Part model, mm, in its own coordinate system. Face numbers are marked on the shaded views. A direction names the side the tool comes from. Give positions to 0.01 mm unless a question says otherwise; leave off trailing zeros. Write each loop counter-clockwise with the first axis right and the second up, starting at its lowest first coordinate (ties: lowest second). Pieces come first, ordered by that corner, then holes. Notation, with made-up numbers: (8.5, 56.25) - (22.5, 56.25) arc R16 ccw to (22.5, 69.25) - close; hole circle Ø10 at (-18, 9.5). An arc over 180 degrees is marked (long way). Answer in a Markdown table with one row per item. Add a question column.
1. Band-saw the part on B-B on x = -50.5. Write the cut outline in (y, z).
2. Band-saw the part on A-A on z = 4.2. State how many separate pieces and enclosed holes the cut face has, plus the area to 3 significant figures.
3. Probe line 1 along X through (y, z) = (45.5, 4.55); line 2 along Y through (x, z) = (-48.5, 2.4); line 3 along X through (y, z) = (34.25, 3.75). List the from-to ranges inside material, lowest first.
4. Drop flat-ended pins along their axis: pin 1 Ø2 at (y, z) = (30, 3) entering from -X; pin 2 Ø1.7 at (y, z) = (36, 2.5) entering from -X; pin 3 Ø1.8 at (x, z) = (-39, 2.5) entering from -Y. Give the stop position or say it passes through.
5. Pull direction Y, two halves, no side cores. Call the marked faces 5, 6 and 7: released by +Y, released by -Y, zero draft, split by the parting line, or undercut.
6. Band-saw the part on C-C on y = 44.5. Write the cut outline in (x, z).
7. Which spindle directions (+Z, -Z, +X, -X, +Y, -Y) get a long thin tool onto all of the face, cutting with end or side? Do the marked faces 1, 2, 3 and 4. Say none if no direction does.
8. Band-saw the part on D-D on x = -62. Write the cut outline in (y, z).
```python
from build123d import *

# Parameters (mm, degrees)
SKETCH2_W           = 40
SKETCH2_H           = 5
SKETCH2_R           = 10
BOSS_EXTRUDE2_DEPTH = 6
FILLET1_R           = 1
FILLET2_R           = 1
FILLET3_R           = 1


with BuildPart() as part:
    # Sketch2 → Boss-Extrude2 (new body)
    # profile 1 of 3: a face of its own
    with BuildSketch(Plane.XY):
        with BuildLine():
            ThreePointArc((-64.563103681, 49.969328221), (-53.382763794, 24.969328221), (-42.202423906, 49.969328221))
            Line((-42.202423906, 49.969328221), (-53.382763794, 49.969328221))
            Line((-53.382763794, 49.969328221), (-64.563103681, 49.969328221))
        make_face()
        with BuildLine():
            ThreePointArc((-43.382763794, 39.969328221), (-60.453831606, 32.89826041), (-53.382763794, 49.969328221))
            ThreePointArc((-53.382763794, 49.969328221), (-46.311695982, 47.040396033), (-43.382763794, 39.969328221))
        make_face(mode=Mode.SUBTRACT)
    # profile 2 of 3: a face of its own
    with BuildSketch(Plane.XY):
        with Locations((-53.382763794, 52.469328221)):
            Rectangle(SKETCH2_W, SKETCH2_H)
    # profile 3 of 3: a face of its own
    with BuildSketch(Plane.XY):
        with Locations((-53.382763794, 39.969328221)):
            Circle(SKETCH2_R)
        with BuildLine():
            ThreePointArc((-52.266628854, 33.05888375), (-48.433016326, 35.019580753), (-46.472319322, 38.853193281))
            Line((-46.472319322, 38.853193281), (-52.266628854, 38.853193281))
            Line((-52.266628854, 38.853193281), (-52.266628854, 33.05888375))
        make_face(mode=Mode.SUBTRACT)
        with BuildLine():
            ThreePointArc((-60.293208266, 38.853193281), (-58.332511262, 35.019580753), (-54.498898734, 33.05888375))
            Line((-54.498898734, 33.05888375), (-54.498898734, 38.853193281))
            Line((-54.498898734, 38.853193281), (-60.293208266, 38.853193281))
        make_face(mode=Mode.SUBTRACT)
        with BuildLine():
            ThreePointArc((-46.472319322, 41.085463162), (-48.433016326, 44.91907569), (-52.266628854, 46.879772693))
            Line((-52.266628854, 46.879772693), (-52.266628854, 41.085463162))
            Line((-52.266628854, 41.085463162), (-46.472319322, 41.085463162))
        make_face(mode=Mode.SUBTRACT)
        with BuildLine():
            ThreePointArc((-54.498898734, 46.879772693), (-58.332511262, 44.91907569), (-60.293208266, 41.085463162))
            Line((-60.293208266, 41.085463162), (-54.498898734, 41.085463162))
            Line((-54.498898734, 41.085463162), (-54.498898734, 46.879772693))
        make_face(mode=Mode.SUBTRACT)
    extrude(amount=BOSS_EXTRUDE2_DEPTH)

    # Fillet1
    fillet1_edges = [part.edges().sort_by_distance(p)[0] for p in [
        (-60.293208266, 41.085463162, 3),
        (-54.498898734, 41.085463162, 3),
        (-54.498898734, 46.879772693, 3),
        (-52.266628854, 46.879772693, 3),
        (-52.266628854, 41.085463162, 3),
        (-46.472319322, 41.085463162, 3),
        (-54.498898734, 33.05888375, 3),
        (-60.293208266, 38.853193281, 3),
        (-46.472319322, 38.853193281, 3),
        (-52.266628854, 33.05888375, 3),
    ]]
    fillet(fillet1_edges, radius=FILLET1_R)

    # Fillet2
    fillet2_edges = [part.edges().sort_by_distance(p)[0] for p in [
        (-54.498898734, 38.853193281, 3),
        (-52.266628854, 38.853193281, 3),
    ]]
    fillet(fillet2_edges, radius=FILLET2_R)

    # Fillet3
    fillet3_edges = [part.edges().sort_by_distance(p)[0] for p in [
        (-73.382763794, 49.969328221, 3),
        (-73.382763794, 54.969328221, 3),
        (-33.382763794, 54.969328221, 3),
        (-33.382763794, 49.969328221, 3),
    ]]
    fillet(fillet3_edges, radius=FILLET3_R)


solid = part.part
```
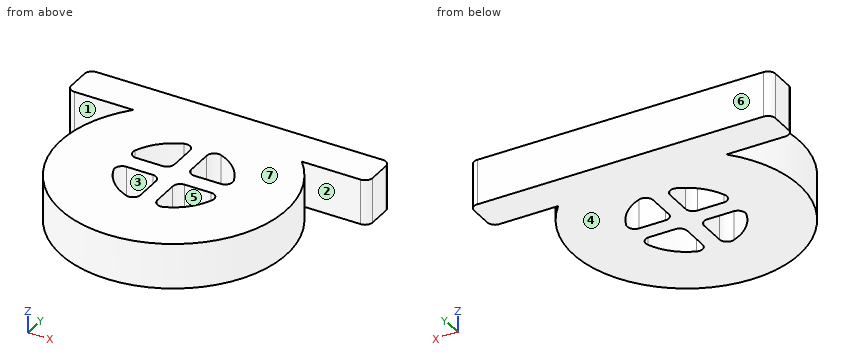
Values:
| question | item | result |
|---|---|---|
| 1 | outline | (25.25, 0) - (33.59, 0) - (33.59, 6) - (25.25, 6) - close; (38.85, 0) - (41.09, 0) - (41.09, 6) - (38.85, 6) - close; (46.35, 0) - (54.97, 0) - (54.97, 6) - (46.35, 6) - close |
| 2 | separate pieces | 1 |
| 2 | enclosed holes | 4 |
| 2 | area | 736 mm² |
| 3 | line 1 | x = -67.33 to -57.67, -54.5 to -52.27, -49.09 to -39.44 |
| 3 | line 2 | y = 25.79 to 34.95, 38.85 to 41.09, 44.99 to 54.97 |
| 3 | line 3 | x = -67.25 to -57.42, -54.5 to -52.26, -49.35 to -39.52 |
| 4 | pin 1 | stops at x = -65.41 |
| 4 | pin 2 | stops at x = -68.05 |
| 4 | pin 3 | stops at y = 33.4 |
| 5 | face 5 | undercut |
| 5 | face 6 | released by +Y |
| 5 | face 7 | zero draft |
| 6 | outline | (-67.68, 0) - (-58.72, 0) - (-58.72, 6) - (-67.68, 6) - close; (-54.5, 0) - (-52.27, 0) - (-52.27, 6) - (-54.5, 6) - close; (-48.05, 0) - (-39.08, 0) - (-39.08, 6) - (-48.05, 6) - close |
| 7 | face 1 | +Z, -Z, -X |
| 7 | face 2 | +Z, -Z, +X |
| 7 | face 3 | +Z, -Z |
| 7 | face 4 | -Z, +X, -X, +Y, -Y |
| 8 | outline | (27.69, 0) - (54.97, 0) - (54.97, 6) - (27.69, 6) - close |
